Here's the drawing with two shaded views (mm, measured from the low corner). I have some questions. A direction names the side the tool comes from. Give positions to 0.01 mm unless a question says otherwise; leave off trailing zeros. Loops run counter-clockwise (first coordinate to the right, second up) from the corner with the lowest first, then second, coordinate; pieces in that order, holes last. Notation, with made-up numbers: (9.25, -23) -> (14.25, -23) arc R19 ccw to (14.25, -7) -> close; hole circle Ø3 at (-25.75, 25). An arc over 180 degrees is marked (long way). Answer in a Markdown table with one row per item. Add a question column.
Item 1: If we section it at B-B (z = 4.5): Write out the boundary of the cut face in (x, y).
Item 2: Which directions (+Z, -Z, +X, -X, +Y, -Y) give clear straight access to the entire face, cutting with the end or side of a thin tool? Please do the marked faces 1, 2, 3, 4 and 5.
Item 3: If we section it at D-D (y = 27): Write out the boundary of the cut face in (x, z).
Item 4: If I drill on line 1 (Y direction, x = 12, z = 22.5); line 2 (X direction, y = 25, z = 7); line 3 (Y direction, x = 60.5, z = 5), over which ranges is the centre line in solid material (lowest first)?
Item 5: If we section it at A-A (y = 9.5): Write out the boundary of the cut face in (x, z), then the cut area to 3 significant figures.
Item 6: If we section it at C-C (x = 24.5): Write out the boundary of the cut face in (y, z).
Item 7: For P1, Ø4, axis at y = 26.5, z = 8.5, coming from the -X side; P2, Ø6.5, axis at x = 40.5, z = 7.5, coming from the -Y side; P3, Ø6, axis at y = 23, z = 26, coming from the +X side, each with a flat end and sliding along its axis, tell me the tip position at first contact or that it passes through.
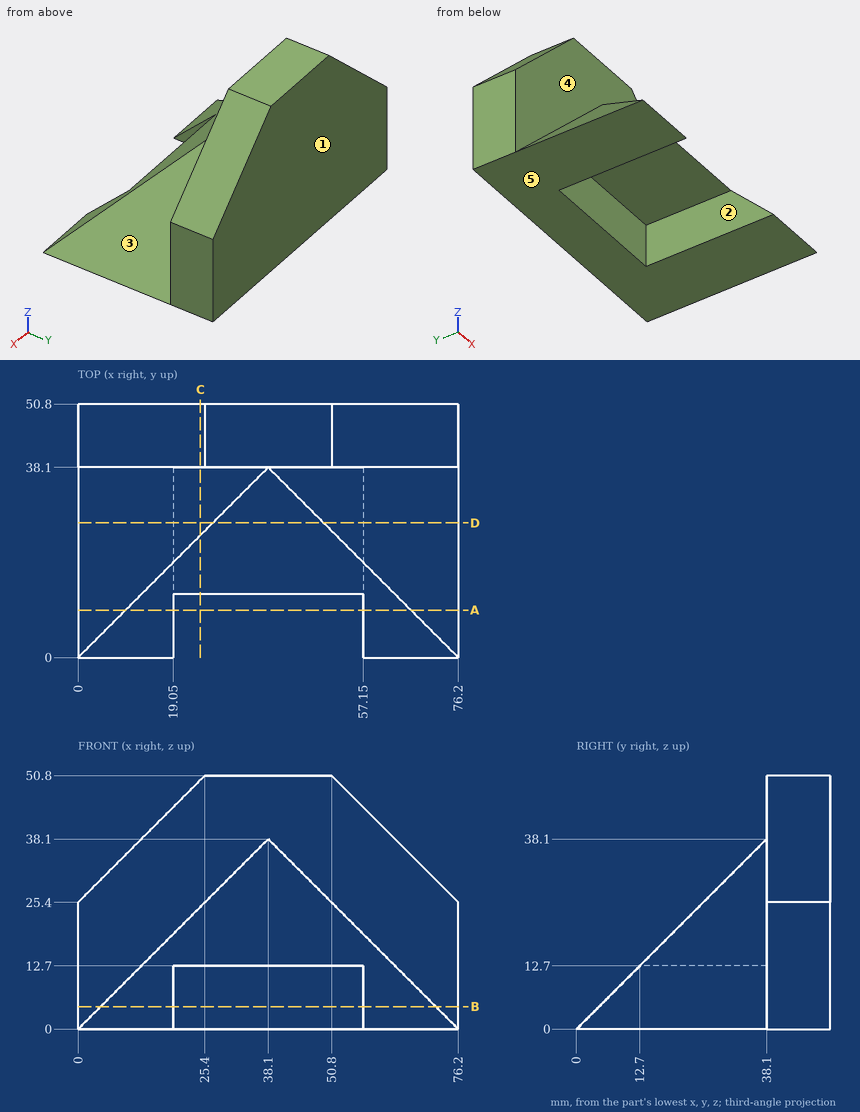
Recorded:
| question | item | result |
|---|---|---|
| 1 | outline | (0, 38.1) -> (4.5, 38.1) -> (4.5, 4.5) -> (19.05, 4.5) -> (19.05, 38.1) -> (57.15, 38.1) -> (57.15, 4.5) -> (71.7, 4.5) -> (71.7, 38.1) -> (76.2, 38.1) -> (76.2, 50.8) -> (0, 50.8) -> close |
| 2 | face 1 | +Z, -Z, +X, -X, +Y |
| 2 | face 2 | -Z, -Y |
| 2 | face 3 | +Z, +X, -Y |
| 2 | face 4 | +Z, -Y |
| 2 | face 5 | -Z, +X, -X, +Y, -Y |
| 3 | outline | (0, 0) -> (19.05, 0) -> (19.05, 12.7) -> (57.15, 12.7) -> (57.15, 0) -> (76.2, 0) -> (49.2, 27) -> (27, 27) -> close |
| 4 | line 1 | y = 38.1 to 50.8 |
| 4 | line 2 | x = 7 to 19.05, 57.15 to 69.2 |
| 4 | line 3 | y = 5 to 50.8 |
| 5 | outline | (0, 0) -> (19.05, 0) -> (19.05, 9.5) -> (9.5, 9.5) -> close; (57.15, 0) -> (76.2, 0) -> (66.7, 9.5) -> (57.15, 9.5) -> close |
| 5 | area | 272 mm^2 |
| 6 | outline | (12.7, 12.7) -> (38.1, 12.7) -> (38.1, 0) -> (50.8, 0) -> (50.8, 49.9) -> (38.1, 49.9) -> (38.1, 24.5) -> (24.5, 24.5) -> close |
| 7 | P1 | stops at x = 6.5 |
| 7 | P2 | stops at y = 38.1 |
| 7 | P3 | stops at x = 53.2 |
